```python
from build123d import *

# Parameters (mm, degrees)
F1_DEPTH = 68.58
F3_DEPTH = 25.4
F4_DEPTH = 10.16
F5_R     = 7.4183703621
F6_DEPTH = 127


with BuildPart() as f1:
    # F0 (on Front) → F1 (new body)
    with BuildSketch(Plane.XZ):
        Polygon((-76.1927291751, 0), (0, 0), (-27.3316595703, 41.0738363862), (-75.8873522282, 41.0738363862), align=None)
    extrude(amount=F1_DEPTH)

    # F2 (on Front) → F3 (join)
    with BuildSketch(Plane.XZ):
        Polygon((-18.7361260581, 55.9061877429), (-76.2327313423, 55.9061877429), (-76.2327313423, 41.2422679365), (-76.3068795204, 0), (0, 0), (16.7718548328, 0), align=None)
    extrude(amount=F3_DEPTH)

    # F4 (add): a face of the model
    f4_faces = [f1.faces().sort_by_distance(p)[0] for p in [
        (-44.3539801272, -68.58, 19.0203203617),
    ]]
    extrude(f4_faces, amount=F4_DEPTH)

    # F5 (on face) → F6 (cut)
    with BuildSketch(Plane(origin=(-76.1885177267, 0, 0.5664485955), x_dir=(0, -1, 0), z_dir=(-0.9999723628, 0, 0.0074346234))):
        with Locations((52.3121915758, 20.9668856114)):
            Circle(F5_R)
    extrude(amount=-F6_DEPTH, mode=Mode.SUBTRACT)


solid = f1.part
```
The listing builds one solid part. Answer for the finished solid, in the listing's coordinates (mm). A direction names the side the tool comes from. Round coordinates to 2 decimals unless told otherwise and drop trailing zeros. Write each loop counter-clockwise with the first axis right and the second up, starting at its lowest first coordinate (ties: lowest second). Pieces come first, ordered by that corner, then holes. Notation, with made-up numbers: (89, 70) -> (130, 70) arc R33 ccw to (130, 104) -> close; hole circle Ø6 at (60, 47). An arc over 180 degrees is marked (long way). Answer as a JSON object with one key per item and string values. Group by question number.
Q1. Section D-D (z = 8) is taken. Write down the section's boundary in (x, y).
Q2. Section B-B (x = 4) is taken. Write down the section's boundary in (y, z).
Q3. Straight lines are drawn through the part: line 1 along Y through (x, z) = (-17, 33); line 2 along Z through (x, y) = (-41.5, -27); line 3 along Y through (x, z) = (-25, 15). For each, find the intervals that lie inside material, in ascending order.
Q4. Each of these flat-tipped pins is pushed along its axis until it touches: pin 1 Ø12 at (x, y) = (-63.5, -64) entering from +Z; pin 2 Ø10 at (x, y) = (3, -32.5) entering from +Z; pin 3 Ø6 at (x, z) = (-42.5, 46.5) entering from -Y. Where does it stop, or does it pass through?
Q5. Section A-A (z = 38.5) is taken. Write down the section's boundary in (x, y), plus the area to 3 significant figures.
Q6. Which of the six approach directions +Z, -Z, +X, -X, +Y, -Y give full straight-line access (tool end or side, diameter ignored) to faces 4 (the face through (-41, -39, 0)), 5 (the face through (-51, -52, 41.074)), 6 (the face through (-10.44, -45.77, 15.69))?
Q7. Determine the mould class of faces 1 (the face through (-42.98, -55.74, 14.71)), 2 (the face through (-0.734, -12.522, 27.562)), 3 (the face through (-76.233, -13, 49)) for opening direction Z: pulls with the +Z half, pulls with the -Z half, needs draft (parallel to the pull), parting line crosses it, or undercut.
Q8. Section C-C (y = -32.5) is taken. Write down the section's boundary in (x, z), plus the area to 3 significant figures.
Check values:
{
 "1": {"outline": "(-76.29, -25.4) -> (-76.13, -25.4) -> (-76.13, -78.74) -> (-5.32, -78.74) -> (-5.32, -25.4) -> (11.69, -25.4) -> (11.69, 0) -> (-76.29, 0) -> close"},
 "2": {"outline": "(-25.4, 0) -> (0, 0) -> (0, 20.11) -> (-25.4, 20.11) -> close"},
 "3": {"line 1": "-25.4 to 0", "line 2": "0 to 41.07", "line 3": "-78.74 to -56.46, -48.17 to 0"},
 "4": {"pin 1": "z = 41.07", "pin 2": "z = 3.01", "pin 3": "y = -25.4"},
 "5": {"outline": "(-76.24, -25.4) -> (-75.91, -25.4) -> (-75.91, -78.74) -> (-25.62, -78.74) -> (-25.62, -25.4) -> (-7.68, -25.4) -> (-7.68, 0) -> (-76.24, 0) -> close", "area": "4,420 mm^2"},
 "6": {"face 4": "-Z, +X, -X, +Y, -Y", "face 5": "+Z, +X, -X, -Y", "face 6": "+Z, +X, -Y"},
 "7": {"face 1": "undercut", "face 2": "pulls with the +Z half", "face 3": "needs draft"},
 "8": {"outline": "(-76.19, 0) -> (0, 0) -> (-27.33, 41.07) -> (-75.89, 41.07) -> close", "area": "2,560 mm^2"}
}
